```python
from build123d import *

# Parameters (mm, degrees)
F1_DEPTH = 10
F2_DEPTH = 17
F3_W     = 100
F3_H     = 35
F4_DEPTH = 3
F5_SIZE2 = 99.99999
F5_SIZE  = 7.49999
F6_SIZE2 = 9.99999
F6_SIZE  = 99.99999
F7_R     = 8
F9_DEPTH = 7
F10_W    = 5.1550631039
F10_H    = 7


# Not quite as in the source:
# - a fillet or chamfer is up to 0.001 mm smaller than in the source, because OpenCascade refuses the exact size
# - a feature of the source that left no trace in its solid (it failed there, or was rolled back) is left out


with BuildPart() as f1:
    # F0 (on Top) → F1 (new body)
    with BuildSketch(Plane.XY):
        Polygon((-58.5, -8.5), (-58.5, -2.5), (-58.5, 0), (-58.5, 2.5), (-58.5, 8.5), (-63.5, 0), align=None)
        Polygon((-58.5, -2.5), (-55, -2.5), (-55, 2.5), (-58.5, 2.5), (-58.5, 0), align=None)
    extrude(amount=F1_DEPTH)

    # F0 (on Top) → F2 (join)
    with BuildSketch(Plane.XY):
        Polygon((-55, -17.5), (55, -17.5), (55, 17.5), (-55, 17.5), (-55, 2.5), (-55, -2.5), align=None)
    extrude(amount=F2_DEPTH)

    # F3 (on face) → F4 (join)
    with BuildSketch(Plane.XY.offset(17)):
        with Locations((5, 0)):
            Rectangle(F3_W, F3_H)
    extrude(amount=F4_DEPTH)

    # F5 (size 7.5 and 100 in the source; OpenCascade refuses exactly that, so slightly less here)
    f5_edges = [f1.edges().sort_by_distance(p)[0] for p in [
        (55, -17.5, 10),
        (55, 17.5, 10),
    ]]
    f5_side = f1.faces().sort_by_distance((55, 0, 10))[0]
    chamfer(f5_edges, length=F5_SIZE, length2=F5_SIZE2, reference=f5_side)

    # F6 (size 100 and 10 in the source; OpenCascade refuses exactly that, so slightly less here)
    f6_edges = [f1.edges().sort_by_distance(p)[0] for p in [
        (55, 0, 20),
    ]]
    chamfer(f6_edges, length=F6_SIZE, length2=F6_SIZE2)

    # F7
    f7_edges = [f1.edges().sort_by_distance(p)[0] for p in [
        (55, -10.00001, 5.000005),
        (55, 10.00001, 5.000005),
    ]]
    fillet(f7_edges, radius=F7_R)

    # F8 (on face) → F9 (join)
    with BuildSketch(Plane.XY):
        with BuildLine():
            ThreePointArc((118.6121593217, 42.5), (89.7807277981, 72.2473973087), (50.3125, 84.8338219329))
            ThreePointArc((50.3125, 84.8338219329), (46.5767340156, 83.4879420476), (45, 79.8435971134))
            Line((45, 79.8435971134), (45, 0))
            Line((45, 0), (50, 2.8867513459))
            Line((50, 2.8867513459), (50, 74.3303437366))
            ThreePointArc((50, 74.3303437366), (51.708597057, 78.0942070001), (55.6666666667, 79.2856999857))
            ThreePointArc((55.6666666667, 79.2856999857), (89.5397594579, 66.4545696505), (114.2820323028, 40))
            Line((114.2820323028, 40), (118.6121593217, 42.5))
        make_face()
        with BuildLine():
            ThreePointArc((120.9846922835, 38.0962798523), (119.8308271392, 40.3155963576), (118.6121593217, 42.5))
            Line((118.6121593217, 42.5), (114.2820323028, 40))
            ThreePointArc((114.2820323028, 40), (115.4987732023, 37.8143223789), (116.6465834297, 35.5916715378))
            Line((116.6465834297, 35.5916715378), (120.9846922835, 38.0962798523))
        make_face()
        with BuildLine():
            ThreePointArc((120.9846922835, -38.0962798523), (130, 0), (120.9846922835, 38.0962798523))
            Line((120.9846922835, 38.0962798523), (116.6465834297, 35.5916715378))
            ThreePointArc((116.6465834297, 35.5916715378), (125, 0), (116.6465834297, -35.5916715378))
            Line((116.6465834297, -35.5916715378), (120.9846922835, -38.0962798523))
        make_face()
        with BuildLine():
            Line((50, -2.8867513459), (45, 0))
            Line((45, 0), (45, -79.8435971134))
            ThreePointArc((45, -79.8435971134), (46.5767340156, -83.4879420476), (50.3125, -84.8338219329))
            ThreePointArc((50.3125, -84.8338219329), (89.7807277981, -72.2473973087), (118.6121593217, -42.5))
            Line((118.6121593217, -42.5), (114.2820323028, -40))
            ThreePointArc((114.2820323028, -40), (89.5397594579, -66.4545696505), (55.6666666667, -79.2856999857))
            ThreePointArc((55.6666666667, -79.2856999857), (51.708597057, -78.0942070001), (50, -74.3303437366))
            Line((50, -74.3303437366), (50, -2.8867513459))
        make_face()
        Polygon((50, 2.8867513459), (45, 0), (50, -2.8867513459), align=None)
        with BuildLine():
            ThreePointArc((118.6121593217, -42.5), (119.8308271392, -40.3155963576), (120.9846922835, -38.0962798523))
            Line((120.9846922835, -38.0962798523), (116.6465834297, -35.5916715378))
            ThreePointArc((116.6465834297, -35.5916715378), (115.4987732023, -37.8143223789), (114.2820323028, -40))
            Line((114.2820323028, -40), (118.6121593217, -42.5))
        make_face()
    extrude(amount=F9_DEPTH)

    # F10 (on face) → F11 (join, up to the next surface of F1)
    with BuildSketch(Plane.YZ.offset(55)):
        with Locations((0, 3.5)):
            Rectangle(F10_W, F10_H)
    extrude(until=Until.NEXT)


solid = f1.part
```
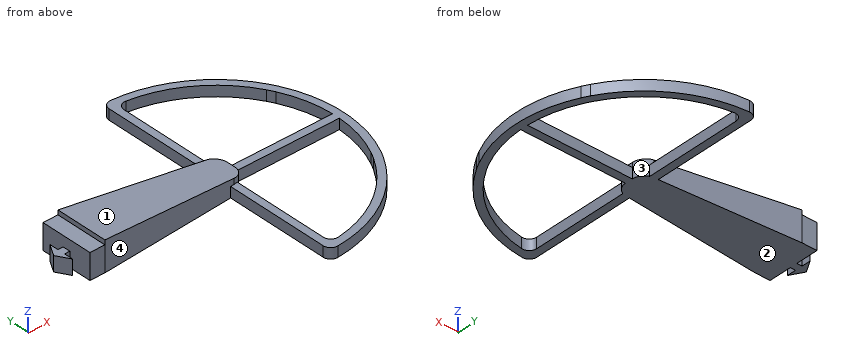
Can you work these out from the model? Positions are in its coordinate system, mm. Face numbers are marked on the shaded views. Round coordinates to 2 decimals unless told otherwise and drop trailing zeros. Loops run counter-clockwise (first coordinate to the right, second up) from the corner with the lowest first, then second, coordinate; pieces in that order, holes last.
Item 1: Please list where these lines run through material, in increasing order: L1, parallel to Y at x = 58, z = 6; L2, parallel to Y at x = -47, z = 15.5; L3, parallel to X at y = -69.5, z = 5.
Item 2: If we mould it in two halves opening along X, with no side actions, what happens to the marked faces 1, 2, 3 and 4? For each: +X half, -X half, draft (parallel to the pull), parting line (faces both ways), or undercut.
Item 3: Suppose I cut it at C-C, the plane x = 75. Write out the boundary of the cut face in (y, z).
Item 4: Suppose I cut it at B-B, the plane y = -5.5. State how many separate pieces and enclosed holes the cut face has, then the cut area to 3 significant figures.
Item 5: Suppose I cut it at D-D, the plane x = -52. Write out the boundary of the cut face in (y, z).
Item 6: Will these pins go through, and if not, where does the flat tip stop? pin 1 Ø1.8 at (y, z) = (4, 5.5) entering from +X; pin 2 Ø1.8 at (x, z) = (-57, 7) entering from -Y; pin 3 Ø6 at (x, z) = (-7, 6.5) entering from +Y (3 decimals); pin 4 Ø6 at (x, y) = (54.5, 43) entering from -Z.
Item 7: Suppose I cut it at A-A, the plane y = -23.5. Write out the boundary of the cut face in (x, z), then the cut area to 3 significant figures.
Reported:
1. L1: y = -84 to -78.94, -2.58 to 2.58, 78.94 to 84
1. L2: y = -17.5 to 17.5
1. L3: x = 45 to 50, 84.62 to 93.94
2. face 1: +X half
2. face 2: draft
2. face 3: undercut
2. face 4: undercut
3. outline: (-79.53, 0) - (-74.16, 0) - (-74.16, 7) - (-79.53, 7) - close; (-2.58, 0) - (2.58, 0) - (2.58, 7) - (-2.58, 7) - close; (74.16, 0) - (79.53, 0) - (79.53, 7) - (74.16, 7) - close
4. separate pieces: 3
4. enclosed holes: 0
4. area: 1,720 mm2
5. outline: (-17.5, 0) - (17.5, 0) - (17.5, 17) - (-17.5, 17) - close
6. pin 1: stops at x = 129.94
6. pin 2: stops at y = -2.5
6. pin 3: stops at y = 14.875
6. pin 4: passes through
7. outline: (45, 0) - (50, 0) - (50, 7) - (45, 7) - close; (121.47, 0) - (126.69, 0) - (126.69, 7) - (121.47, 7) - close
7. area: 71.5 mm2
